Build history of the part. All positions in model axes, mm. Give positions to 0.01 mm unless a question says otherwise; leave off trailing zeros. Loops run counter-clockwise (first coordinate to the right, second up) from the corner with the lowest first, then second, coordinate; pieces in that order, holes last. Notation, with made-up numbers: M -35.5,-38.5 L -23.5,-38.5 A37 ccw -23.5,-0.5 Z; hole C 18,1.25 d5. An arc over 180 degrees is marked long. Put each result on its own line as item: value.
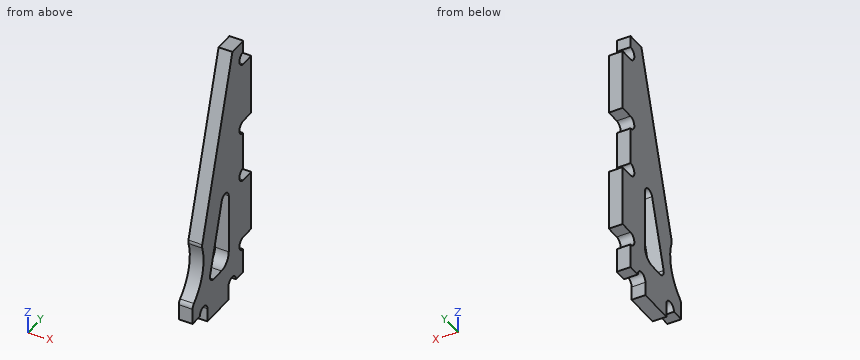
```python
from build123d import *

# Parameters (mm, degrees)
EXTRUDE_1_DEPTH = 2.2
FILLET_1_R      = 2
FILLET_2_R      = 1


with BuildPart() as part:
    # 草图1 → 凸台-拉伸1 (new body)
    with BuildSketch(Plane(origin=(0, 0, 0), x_dir=(0, 0, -1), z_dir=(1, 0, 0))):
        with BuildLine():
            ThreePointArc((7, -1.1), (5.95, -2.15), (4.9, -1.1))
            Line((4.9, -1.1), (4.9, 1.1))
            Line((4.9, 1.1), (-4.9, 1.1))
            Line((-4.9, 1.1), (-4.9, -1.1))
            ThreePointArc((-4.9, -1.1), (-5.95, -2.15), (-7, -1.1))
            Line((-7, -1.1), (-13, -1.1))
            ThreePointArc((-13, -1.1), (-14.05, -2.15), (-15.1, -1.1))
            Line((-15.1, -1.1), (-15.1, 1.1))
            Line((-15.1, 1.1), (-24.9, 1.1))
            Line((-24.9, 1.1), (-24.9, -1.1))
            ThreePointArc((-24.9, -1.1), (-25.95, -2.15), (-27, -1.1))
            Line((-27, -1.1), (-28.9, -1.1))
            Line((-28.9, -1.1), (-28.9, -4.1))
            Line((-28.9, -4.1), (-0.723011959, -12.522469251))
            ThreePointArc((-0.723011959, -12.522469251), (4.018082479, -12.374065966), (7.9, -15.1))
            Line((7.9, -15.1), (10.9, -15.1))
            Line((10.9, -15.1), (10.9, -13.1))
            ThreePointArc((10.9, -13.1), (9.85, -12.05), (10.9, -11))
            Line((10.9, -11), (13.1, -11))
            Line((13.1, -11), (13.1, -5.2))
            Line((13.1, -5.2), (10.9, -5.2))
            ThreePointArc((10.9, -5.2), (9.85, -4.15), (10.9, -3.1))
            Line((10.9, -3.1), (10.9, -1.1))
            Line((10.9, -1.1), (7, -1.1))
        make_face()
        Polygon((6.9, -10.626211615), (-11.587689765, -5.1), (6.9, -5.1), align=None, mode=Mode.SUBTRACT)
    extrude(amount=EXTRUDE_1_DEPTH)

    # 圆角1
    fillet_1_edges = [part.edges().sort_by_distance(p)[0] for p in [
        (1.1, -5.1, -6.9),
    ]]
    fillet(fillet_1_edges, radius=FILLET_1_R)

    # 圆角2
    fillet_2_edges = [part.edges().sort_by_distance(p)[0] for p in [
        (1.1, -5.1, 11.587689765),
        (1.1, -10.626211615, -6.9),
        (1.1, -12.522469251, 0.723011959),
        (1.1, -15.1, -7.9),
    ]]
    fillet(fillet_2_edges, radius=FILLET_2_R)


solid = part.part
```
Q1. Probe line 1 (Z direction, x = 0.25, y = -2.75); line 2 (Y direction, x = 1, z = -9); line 3 (Y direction, x = 0.9, z = -4). List the from-to ranges inside material, lowest first. Write a range as from..to.
Here are the results:
line 1: -10.9..28.9
line 2: -15.1..-1.1
line 3: -12.37..-9.76, -5.1..1.1
Q2. Slice it at D-D (z = 14.05). List the corners of the cut face in (x, y).
Here are the results:
outline: M 0,-8.54 L 2.2,-8.54 L 2.2,-2.15 L 0,-2.15 Z
Q3. Slice it at C-C (z = 0). List the corners of the cut face in (x, y), and give its area (3 significant figures).
Here are the results:
outline: M 0,-12.3 L 2.2,-12.3 L 2.2,-8.56 L 0,-8.56 Z; M 0,-5.1 L 2.2,-5.1 L 2.2,1.1 L 0,1.1 Z
area: 21.9 mm²
Q4. Drop flat-ended pins along their axis: pin 1 Ø1.1 at (x, z) = (1, -12) entering from +Y; pin 2 Ø2 at (y, z) = (-2.5, 2.5) entering from -X; pin 3 Ø0.7 at (x, z) = (0.5, -11.5) entering from -Y; pin 4 Ø1 at (x, z) = (1, 7) entering from +Y. Give the stop position or say it passes through.
Here are the results:
pin 1: y = -5.2
pin 2: x = 0
pin 3: y = -11
pin 4: y = -1.1
Q5. Slice it at A-A (y = -0.25). List the corners of the cut face in (x, z), and give its area (3 significant figures).
Here are the results:
outline: M 0,-4.9 L 2.2,-4.9 L 2.2,4.9 L 0,4.9 Z; M 0,15.1 L 2.2,15.1 L 2.2,24.9 L 0,24.9 Z
area: 43.1 mm²
